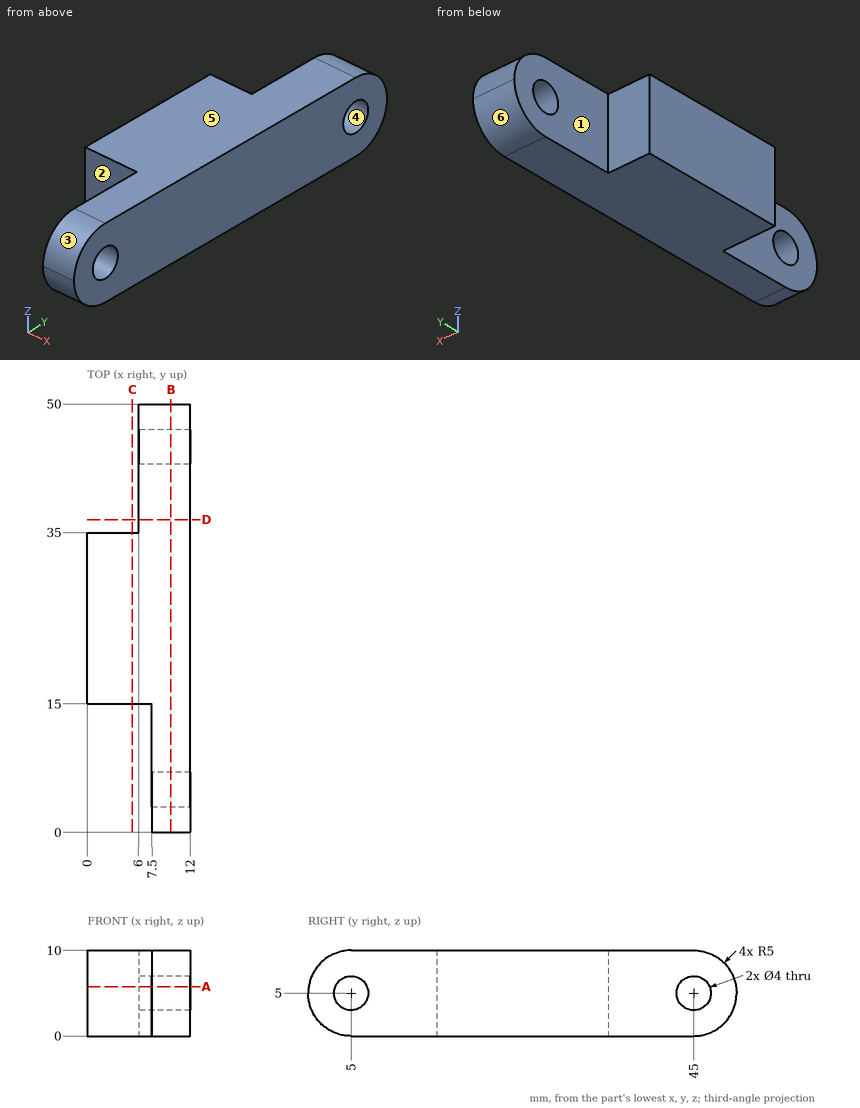
Could you check a few things on this drawing? It's one solid part, dimensions in mm from its lowest x, y, z. A direction names the side the tool comes from. Coordinates: 2 decimals unless noted, no trailing zeros. Order: outer loops, then holes, each group sorted by start corner. A loop starts at its lowest first (then second) coordinate and runs counter-clockwise, first axis right, second up. Notation, with made-up numbers: M -28,26.5 L 16,26.5 A16 ccw 16,34.5 Z; hole C 29.5,12 d8. An arc over 180 degrees is marked long. Answer as a JSON object with one key per item and string values. Group by question number.
(1) For pin 1 (3 mm diameter, centred on x = 3, z = 6, fed in from +Y); pin 2 (4.5 mm diameter, centred on y = 45, z = 5, fed in from -X); pin 3 (2 mm diameter, centred on x = 4, z = 7.5, fed in from -Y), each with a flat end and sliding along its axis, tell me the tip position at first contact or that it passes through.
(2) Suppose I cut it at D-D, the plane y = 36.5. Please give me the cut outline in (x, z), then the cut area to 3 significant figures.
(3) Suppose I cut it at A-A, the plane z = 5.75. Please give me the cut outline in (x, y).
(4) Suppose I cut it at C-C, the plane x = 5.25. Please give me the cut outline in (y, z), then the cut area to 3 significant figures.
(5) If we mould it in two halves opening along Y, with no side actions, what happens to the marked faces 4, 5 and 6? For each: released by +Y, released by -Y, zero draft, split by the parting line, or undercut.
(6) I need wall thicknesses on probe 1 along Z at (x, y) = (9.6, 5); probe 2 along Y at (x, z) = (9.5, 5.5) (1 decimal); probe 3 along X at (y, z) = (12.5, 9). Which ranges of each line are inside material? Lowest first, please.
(7) Which directions (+Z, -Z, +X, -X, +Y, -Y) give clear straight access to the entire face, cutting with the end or side of a thin tool? Please do the marked faces 1, 2 and 3.
(8) Suppose I cut it at B-B, the plane x = 9.75. State how many separate pieces and enclosed holes the cut face has, then the cut area to 3 significant figures.
Values found:
{
 "1": {"pin 1": "stops at y = 35", "pin 2": "stops at x = 6", "pin 3": "stops at y = 15"},
 "2": {"outline": "M 6,0 L 12,0 L 12,10 L 6,10 Z", "area": "60.0 mm^2"},
 "3": {"outline": "M 0,15 L 7.5,15 L 7.5,6.85 L 12,6.85 L 12,43.15 L 6,43.15 L 6,35 L 0,35 Z; M 6,46.85 L 12,46.85 L 12,49.94 L 6,49.94 Z; M 7.5,0.06 L 12,0.06 L 12,3.15 L 7.5,3.15 Z"},
 "4": {"outline": "M 15,0 L 35,0 L 35,10 L 15,10 Z", "area": "200 mm^2"},
 "5": {"face 4": "undercut", "face 5": "zero draft", "face 6": "released by +Y"},
 "6": {"probe 1": "z = 0 to 3, 7 to 10", "probe 2": "y = 0 to 3.1, 6.9 to 43.1, 46.9 to 50", "probe 3": "x = 7.5 to 12"},
 "7": {"face 1": "+Z, -Z, -X, +Y", "face 2": "+Z, -Z, -X, -Y", "face 3": "+Z, +X, -X, -Y"},
 "8": {"separate pieces": "1", "enclosed holes": "2", "area": "453 mm^2"}
}
